```python
from build123d import *

# Parameters (mm, degrees)
SKETCH_1_R          = 23
EXTRUDE_1_DEPTH     = 5
FILLET_1_R          = 4
EXTRUDE_2_DEPTH     = 2
CUT_EXTRUDE_3_DEPTH = 45.18427322
SKETCH_7_R          = 14
EXTRUDE_3_DEPTH     = 5
SKETCH_8_R          = 22.5
EXTRUDE_4_DEPTH     = 5


with BuildPart() as part:
    # 草图1 → 凸台-拉伸1 (new body)
    with BuildSketch(Plane.XY):
        Circle(SKETCH_1_R)
    extrude(amount=EXTRUDE_1_DEPTH)

    # 圆角1
    fillet_1_edges = [part.edges().sort_by_distance(p)[0] for p in [
        (-23, 0, 0),
    ]]
    fillet(fillet_1_edges, radius=FILLET_1_R)

    # 草图4 → 凸台-拉伸2 (add)
    with BuildSketch(Plane.XY):
        with BuildLine():
            Line((-31, -26.5), (31, -26.5))
            ThreePointArc((31, -26.5), (33.828427125, -25.328427125), (35, -22.5))
            Line((35, -22.5), (35, 22.5))
            ThreePointArc((35, 22.5), (33.828427125, 25.328427125), (31, 26.5))
            Line((31, 26.5), (-31, 26.5))
            ThreePointArc((-31, 26.5), (-33.828427125, 25.328427125), (-35, 22.5))
            Line((-35, 22.5), (-35, -22.5))
            ThreePointArc((-35, -22.5), (-33.828427125, -25.328427125), (-31, -26.5))
        make_face()
    extrude(amount=EXTRUDE_2_DEPTH)

    # 草图6 → 切除-拉伸3 (cut, through all)
    with BuildSketch(Plane(origin=(0, 0, 0), x_dir=(-1, 0, 0), z_dir=(0, 0, -1))):
        with BuildLine():
            Line((28, 21.5), (25, 21.5))
            ThreePointArc((25, 21.5), (23.5, 20), (25, 18.5))
            Line((25, 18.5), (28, 18.5))
            ThreePointArc((28, 18.5), (29.5, 20), (28, 21.5))
        make_face()
        with BuildLine():
            Line((25, -18.5), (28, -18.5))
            ThreePointArc((28, -18.5), (29.5, -20), (28, -21.5))
            Line((28, -21.5), (25, -21.5))
            ThreePointArc((25, -21.5), (23.5, -20), (25, -18.5))
        make_face()
        with BuildLine():
            Line((-28, -21.5), (-25, -21.5))
            ThreePointArc((-25, -21.5), (-23.5, -20), (-25, -18.5))
            Line((-25, -18.5), (-28, -18.5))
            ThreePointArc((-28, -18.5), (-29.5, -20), (-28, -21.5))
        make_face()
        with BuildLine():
            Line((-28, 21.5), (-25, 21.5))
            ThreePointArc((-25, 21.5), (-23.5, 20), (-25, 18.5))
            Line((-25, 18.5), (-28, 18.5))
            ThreePointArc((-28, 18.5), (-29.5, 20), (-28, 21.5))
        make_face()
    extrude(amount=-CUT_EXTRUDE_3_DEPTH, mode=Mode.SUBTRACT)

    # 草图7 → 凸台-拉伸3 (add)
    with BuildSketch(Plane.XY.offset(5)):
        Circle(SKETCH_7_R)
    extrude(amount=EXTRUDE_3_DEPTH)

    # 草图8 → 凸台-拉伸4 (add)
    with BuildSketch(Plane.XY.offset(10)):
        Circle(SKETCH_8_R)
    extrude(amount=EXTRUDE_4_DEPTH)


solid = part.part
```
The listing builds one solid part. Answer for the finished solid, in the listing's coordinates (mm). A direction names the side the tool comes from. Round coordinates to 2 decimals unless told otherwise and drop trailing zeros. Loops run counter-clockwise (first coordinate to the right, second up) from the corner with the lowest first, then second, coordinate; pieces in that order, holes last.
1) A cutting plane is placed at C-C on x = 0. Determine the outline of the cut face in (y, z).
Outcome:
outline: (-26.5, 0) - (26.5, 0) - (26.5, 2) - (22.46, 2) arc R4 ccw to (23, 4) - (23, 5) - (14, 5) - (14, 10) - (22.5, 10) - (22.5, 15) - (-22.5, 15) - (-22.5, 10) - (-14, 10) - (-14, 5) - (-23, 5) - (-23, 4) arc R4 ccw to (-22.46, 2) - (-26.5, 2) - close
2) A cutting plane is placed at B-B on z = 12.5. Determine the outline of the cut face in (x, y), plus the area to 3 significant figures.
Outcome:
outline: circle Ø45 at (0, 0)
area: 1,590 mm2
3) A cutting plane is placed at A-A on z = 1.25. Determine the outline of the cut face in (x, y).
Outcome:
outline: (-35, -22.5) arc R4 ccw to (-31, -26.5) - (31, -26.5) arc R4 ccw to (35, -22.5) - (35, 22.5) arc R4 ccw to (31, 26.5) - (-31, 26.5) arc R4 ccw to (-35, 22.5) - close; hole (-28, -21.5) - (-25, -21.5) arc R1.5 ccw to (-25, -18.5) - (-28, -18.5) arc R1.5 ccw to start; hole (-28, 18.5) - (-25, 18.5) arc R1.5 ccw to (-25, 21.5) - (-28, 21.5) arc R1.5 ccw to start; hole (25, -21.5) - (28, -21.5) arc R1.5 ccw to (28, -18.5) - (25, -18.5) arc R1.5 ccw to start; hole (25, 18.5) - (28, 18.5) arc R1.5 ccw to (28, 21.5) - (25, 21.5) arc R1.5 ccw to start
4) Consider line 1 (Y direction, x = 27, z = 1.75); line 2 (Z direction, x = 8, y = 22); line 3 (Z direction, x = -15, y = 14.5). Determine where each line is inside the solid, lowest interval first.
Outcome:
line 1: y = -26.5 to -21.5, -18.5 to 18.5, 21.5 to 26.5
line 2: z = 0 to 2
line 3: z = 0 to 5, 10 to 15
5) For faces 4 (the face through (-35, 0, 1)), 5 (the face through (23.5, 20, 1)), 6 (the face through (0, -15, 5)), determine the directions among +Z, -Z, +X, -X, +Y, -Y from which every point of the face is accessible in a straight line to the end or side of a thin tool.
Outcome:
face 4: +Z, -Z, -X, +Y, -Y
face 5: +Z, -Z
face 6: none
6) For a pull along X with two mould halves and no side action, classify faces 1 (the face through (0, 0, 0)), 2 (the face through (-33.859, -25.297, 0.986)), 3 (the face through (23.5, -20, 1)) as released by +X, released by -X, zero draft, split by the parting line, or undercut.
Outcome:
face 1: zero draft
face 2: released by -X
face 3: undercut
7) Given P1, Ø1, axis at x = 11.5, z = 6, coming from the -Y side; P2, Ø6, axis at x = 17, z = 11, coming from the -Y side; P3, Ø6, axis at y = -10, z = 5.5, coming from the +X side, each flat-ended and moving along its own axis, determine where each tip first touches the part or whether it passes through.
Outcome:
P1: stops at y = -8.66
P2: stops at y = -17.61
P3: stops at x = 21.9
8) A cutting plane is placed at D-D on y = -20. Give the number of separate pieces and of enclosed holes in the cut face, plus the area to 3 significant figures.
Outcome:
separate pieces: 4
enclosed holes: 0
area: 286 mm2
